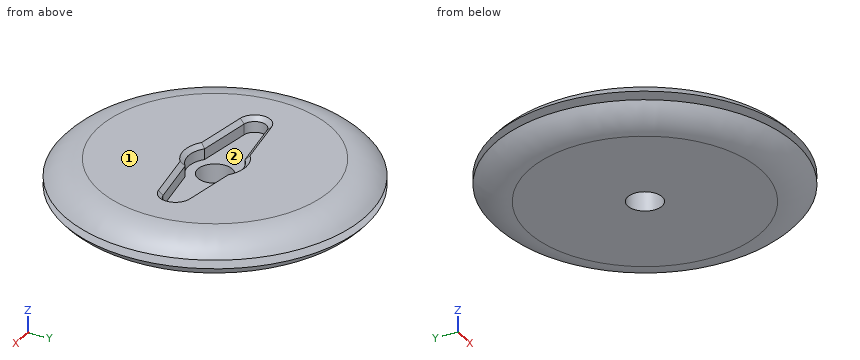
from build123d import *

# Parameters (mm, degrees)
SKETCH_1_R               = 1.5
EXTRUDE_1_DEPTH          = 2.3
SKETCH_2_R               = 4.4
EXTRUDE_2_DEPTH          = 3.2
SKETCH_3_R               = 4.4
SKETCH_3_R_2             = 3.4
SKETCH_3_R_3             = 2.75
SKETCH_3_R_4             = 1.5
CUT_EXTRUDE_1_DEPTH      = 1
BOSS_EXTRUDE1_DEPTH      = 2
BOSS_EXTRUDE1_DEPTH_BACK = 2
SKETCH1_R                = 35
INTERSECT2_OUTLINE_R     = 4.4
INTERSECT2_OUTLINE_R_2   = 3.4
INTERSECT2_OUTLINE_R_3   = 2.75
INTERSECT2_DEPTH         = 5.5
INTERSECT2_START         = 1
INTERSECT2_2_OUTLINE_R   = 4.4
INTERSECT2_2_OUTLINE_R_2 = 3.4
INTERSECT2_2_OUTLINE_R_3 = 2.75
INTERSECT2_2_OUTLINE_R_4 = 1.5
INTERSECT2_2_DEPTH       = 4.5
FILLET1_R                = 10
SKETCH2_R                = 25
BOSS_EXTRUDE2_DEPTH      = 2
SKETCH3_R                = 27
BOSS_EXTRUDE3_DEPTH      = 2
SKETCH4_R                = 6
CUT_EXTRUDE1_DEPTH       = 2
CUT_EXTRUDE3_REACH       = 52.14
SKETCH5_R                = 4
CUT_EXTRUDE4_START       = -2
CUT_EXTRUDE4_DEPTH       = 2
CHAMFER1_SIZE            = 1
CUT_EXTRUDE5_DEPTH       = 1.5


# Read off the part's stored shape, not the designer's step: Intersect2
with BuildPart() as part:
    # Эскиз1 → Бобышка-Вытянуть1 (new body)
    with BuildSketch(Plane.XY):
        with BuildLine():
            Line((-3.968626967, 4.5), (-16.888114198, 2.469689731))
            ThreePointArc((-16.888114198, 2.469689731), (-19, 0), (-16.888114198, -2.469689731))
            Line((-16.888114198, -2.469689731), (-3.968626967, -4.5))
            ThreePointArc((-3.968626967, -4.5), (0, -6), (3.968626967, -4.5))
            Line((3.968626967, -4.5), (16.888114198, -2.469689731))
            ThreePointArc((16.888114198, -2.469689731), (19, 0), (16.888114198, 2.469689731))
            Line((16.888114198, 2.469689731), (3.968626967, 4.5))
            ThreePointArc((3.968626967, 4.5), (0, 6), (-3.968626967, 4.5))
        make_face()
        Circle(SKETCH_1_R, mode=Mode.SUBTRACT)
    extrude(amount=EXTRUDE_1_DEPTH)

    # Эскиз2 → Бобышка-Вытянуть2 (add)
    with BuildSketch(Plane.XY.offset(2.3)):
        with Locations(Location((0, 0, 0), (0, 0, 180))):
            Circle(SKETCH_2_R)
        Polygon((0.333439775, 2.639447604), (0, 3.05), (-0.333439775, 2.639447604), (-0.758504156, 2.954178641), (-0.979368078, 2.473601404), (-1.469348706, 2.672735374), (-1.563759083, 2.15232973), (-2.087868673, 2.223354314), (-2.049893354, 1.695819264), (-2.575200173, 1.634271725), (-2.407225286, 1.132754236), (-2.900722375, 0.942501833), (-2.6133024, 0.498514094), (-3.043981522, 0.191511085), (-2.655176114, -0.167049522), (-2.995976115, -0.571513009), (-2.530215347, -0.822116802), (-2.75972251, -1.298626839), (-2.246271844, -1.42552746), (-2.35006539, -1.944143169), (-1.821186821, -1.939366985), (-1.792745019, -2.467501833), (-1.281669931, -2.33134895), (-1.122779886, -2.835818282), (-0.661621006, -2.576843686), (-0.382266362, -3.025949839), (0, -2.660425857), (0.382266362, -3.025949839), (0.661621006, -2.576843686), (1.122779886, -2.835818282), (1.281669931, -2.33134895), (1.792745019, -2.467501833), (1.821186821, -1.939366985), (2.35006539, -1.944143169), (2.246271844, -1.42552746), (2.75972251, -1.298626839), (2.530215347, -0.822116802), (2.995976115, -0.571513009), (2.655176114, -0.167049522), (3.043981522, 0.191511085), (2.6133024, 0.498514094), (2.900722375, 0.942501833), (2.407225286, 1.132754236), (2.575200173, 1.634271725), (2.049893354, 1.695819264), (2.087868673, 2.223354314), (1.563759083, 2.15232973), (1.469348706, 2.672735374), (0.979368078, 2.473601404), (0.758504156, 2.954178641), align=None, mode=Mode.SUBTRACT)
    extrude(amount=EXTRUDE_2_DEPTH)

    # Эскиз3 → Вырез-Вытянуть1 (cut)
    # profile 1 of 2: a face of its own
    with BuildSketch(Plane(origin=(0, 0, 0), x_dir=(-1, 0, 0), z_dir=(0, 0, -1))):
        Circle(SKETCH_3_R)
        Circle(SKETCH_3_R_2, mode=Mode.SUBTRACT)
    # profile 2 of 2: a face of its own
    with BuildSketch(Plane(origin=(0, 0, 0), x_dir=(-1, 0, 0), z_dir=(0, 0, -1))):
        Circle(SKETCH_3_R_3)
        Circle(SKETCH_3_R_4, mode=Mode.SUBTRACT)
    extrude(amount=-CUT_EXTRUDE_1_DEPTH, mode=Mode.SUBTRACT)


with BuildPart() as body_2:
    # Sketch1 → Boss-Extrude1 (new, two sides: drawn at the far end of the back side and taken through both)
    with BuildSketch(Plane(origin=(0, 0, 0), x_dir=(-1, 0, 0), z_dir=(0, 0, -1)).offset(-BOSS_EXTRUDE1_DEPTH_BACK)):
        Circle(SKETCH1_R)
    extrude(amount=BOSS_EXTRUDE1_DEPTH + BOSS_EXTRUDE1_DEPTH_BACK)


with BuildPart() as intersect2_tool:
    # Intersect2 outline → Intersect2 (new body)
    # profile 1 of 2: a face of its own
    with BuildSketch(Plane.XY):
        with BuildLine():
            ThreePointArc((3.968626967, 4.5), (0, 6), (-3.968626967, 4.5))
            Line((-3.968626967, 4.5), (-16.888114198, 2.469689731))
            ThreePointArc((-16.888114198, 2.469689731), (-19, 0), (-16.888114198, -2.469689731))
            Line((-16.888114198, -2.469689731), (-3.968626967, -4.5))
            ThreePointArc((-3.968626967, -4.5), (0, -6), (3.968626967, -4.5))
            Line((3.968626967, -4.5), (16.888114198, -2.469689731))
            ThreePointArc((16.888114198, -2.469689731), (19, 0), (16.888114198, 2.469689731))
            Line((16.888114198, 2.469689731), (3.968626967, 4.5))
        make_face()
        Circle(INTERSECT2_OUTLINE_R, mode=Mode.SUBTRACT)
    # profile 2 of 2: a face of its own
    with BuildSketch(Plane.XY):
        Circle(INTERSECT2_OUTLINE_R_2)
        Circle(INTERSECT2_OUTLINE_R_3, mode=Mode.SUBTRACT)
    extrude(amount=INTERSECT2_DEPTH)


with BuildPart() as part_1:
    add(part.part)

    # Intersect2: cut by intersect2_tool
    add(intersect2_tool.part, mode=Mode.SUBTRACT)


with BuildPart() as body_2_1:
    add(body_2.part)

    # Intersect2: cut by intersect2_tool
    add(intersect2_tool.part, mode=Mode.SUBTRACT)


with BuildPart() as intersect2_2_tool:
    # Intersect2 2 outline → Intersect2 2 (new body)
    # profile 1 of 2: a face of its own
    with BuildSketch(Plane.XY.offset(INTERSECT2_START)):
        Circle(INTERSECT2_2_OUTLINE_R)
        Circle(INTERSECT2_2_OUTLINE_R_2, mode=Mode.SUBTRACT)
    # profile 2 of 2: a face of its own
    with BuildSketch(Plane.XY.offset(INTERSECT2_START)):
        Circle(INTERSECT2_2_OUTLINE_R_3)
        Circle(INTERSECT2_2_OUTLINE_R_4, mode=Mode.SUBTRACT)
    extrude(amount=INTERSECT2_2_DEPTH)


with BuildPart() as part_2:
    add(part_1.part)

    # Intersect2 2: cut by intersect2_2_tool
    add(intersect2_2_tool.part, mode=Mode.SUBTRACT)


with BuildPart() as body_2_2:
    add(body_2_1.part)

    # Intersect2 2: cut by intersect2_2_tool
    add(intersect2_2_tool.part, mode=Mode.SUBTRACT)

    # Fillet1
    # the kernel refuses this fillet: 10 mm, written as the material it takes off along each edge
    with BuildSketch(Plane(origin=(0, 0, 2), x_dir=(-1, 0, 0), z_dir=(0, -1, 0))) as fillet1_piece_1:
        with BuildLine():
            CenterArc((27, 10), FILLET1_R, 270, 53.130102354)
            Line((27, 0), (27, -0.2))
            Line((27, -0.2), (35, -0.2))
            Line((35, -0.2), (35.2, 0))
            ThreePointArc((35.2, 0), (35.2, 2), (35.16, 3.88))
            Line((35.16, 3.88), (35, 4))
        make_face()
    revolve(axis=Axis((0, 0, 2), (0, 0, -1)), mode=Mode.SUBTRACT)


with BuildPart() as body_2_2_1:
    # Mirror9: mirrored copy
    add(body_2_2.part.mirror(Plane.XY.offset(-3)))


with BuildPart() as body_2_3:
    add(body_2_2.part)

    add(body_2_2_1.part)  # Boss-Extrude2 merges body 2 2
    # Sketch2 → Boss-Extrude2 (add)
    with BuildSketch(Plane(origin=(0, 0, -2), x_dir=(-1, 0, 0), z_dir=(0, 0, -1))):
        Circle(SKETCH2_R)
    extrude(amount=BOSS_EXTRUDE2_DEPTH)

    # Sketch3 → Boss-Extrude3 (add)
    with BuildSketch(Plane(origin=(0, 0, -8), x_dir=(-1, 0, 0), z_dir=(0, 0, -1))):
        Circle(SKETCH3_R)
    extrude(amount=-BOSS_EXTRUDE3_DEPTH)

    # Sketch4 → Cut-Extrude1 (cut)
    with BuildSketch(Plane.XY):
        Circle(SKETCH4_R)
    extrude(amount=CUT_EXTRUDE1_DEPTH, mode=Mode.SUBTRACT)

    # Sketch5 → Cut-Extrude3 (cut, up to next)
    with BuildSketch(Plane.XY, mode=Mode.PRIVATE) as cut_extrude3_sk1:
        Circle(SKETCH5_R)
    cut_extrude3_tool1 = extrude(cut_extrude3_sk1.sketch, amount=-CUT_EXTRUDE3_REACH, mode=Mode.PRIVATE) & body_2_3.part
    add(cut_extrude3_tool1.solids().sort_by_distance((0, 0, 0))[0], mode=Mode.SUBTRACT)

    # Sketch6 → Cut-Extrude4 (cut)
    with BuildSketch(Plane.XY.offset(2).offset(CUT_EXTRUDE4_START)):
        with BuildLine():
            Line((16.919163334, 2.66726491), (4.056712891, 4.68861179))
            ThreePointArc((4.056712891, 4.68861179), (0, 6.2), (-4.056712891, 4.68861179))
            Line((-4.056712891, 4.68861179), (-16.919163334, 2.66726491))
            ThreePointArc((-16.919163334, 2.66726491), (-19.2, 0), (-16.919163334, -2.66726491))
            Line((-16.919163334, -2.66726491), (-4.056712891, -4.68861179))
            ThreePointArc((-4.056712891, -4.68861179), (0, -6.2), (4.056712891, -4.68861179))
            Line((4.056712891, -4.68861179), (16.919163334, -2.66726491))
            ThreePointArc((16.919163334, -2.66726491), (19.2, 0), (16.919163334, 2.66726491))
        make_face()
    extrude(amount=CUT_EXTRUDE4_DEPTH, mode=Mode.SUBTRACT)

    # Chamfer1
    chamfer1_edges = [body_2_3.edges().sort_by_distance(p)[0] for p in [
        (0, 6.2, 2),
        (-10.487938112, 3.67793835, 2),
        (-19.2, 0, 2),
        (-10.487938112, -3.67793835, 2),
        (0, -6.2, 2),
        (10.487938112, -3.67793835, 2),
        (19.2, 0, 2),
        (10.487938112, 3.67793835, 2),
    ]]
    chamfer(chamfer1_edges, length=CHAMFER1_SIZE)

    # Sketch8 → Cut-Extrude5 (cut)
    with BuildSketch(Plane.XY):
        with BuildLine():
            Line((-4.056712891, 4.68861179), (-16.919163334, 2.66726491))
            ThreePointArc((-16.919163334, 2.66726491), (-19.2, 0), (-16.919163334, -2.66726491))
            Line((-16.919163334, -2.66726491), (-4.056712891, -4.68861179))
            ThreePointArc((-4.056712891, -4.68861179), (0, -6.2), (4.056712891, -4.68861179))
            Line((4.056712891, -4.68861179), (16.919163334, -2.66726491))
            ThreePointArc((16.919163334, -2.66726491), (19.2, 0), (16.919163334, 2.66726491))
            Line((16.919163334, 2.66726491), (4.056712891, 4.68861179))
            ThreePointArc((4.056712891, 4.68861179), (0, 6.2), (-4.056712891, 4.68861179))
        make_face()
    extrude(amount=-CUT_EXTRUDE5_DEPTH, mode=Mode.SUBTRACT)


solid = body_2_3.part
Can you work these out from the model? Positions are in its coordinate system, mm. Face numbers are marked on the shaded views. Coordinates: 2 decimals unless noted, no trailing zeros. Write each loop counter-clockwise with the first axis right and the second up, starting at its lowest first coordinate (ties: lowest second). Pieces come first, ordered by that corner, then holes. Notation, with made-up numbers: (83, -9) -> (109, -9) arc R31 cw to (109, 22) -> close; hole circle Ø7 at (36.5, -18). An arc over 180 degrees is marked (long way). Write item = value, one per line.
(1) Imagine slicing it at B-B (x = 0). Please give me the cut outline in (y, z).
Verdict:
outline = (-35, -4) arc R10 ccw to (-27, -8) -> (-4, -8) -> (-4, -1.5) -> (-6.2, -1.5) -> (-6.2, 1) -> (-7.2, 2) -> (-27, 2) arc R10 ccw to (-35, -2) -> (-25, -2) -> (-25, -4) -> close; (4, -8) -> (27, -8) arc R10 ccw to (35, -4) -> (25, -4) -> (25, -2) -> (35, -2) arc R10 ccw to (27, 2) -> (7.2, 2) -> (6.2, 1) -> (6.2, -1.5) -> (4, -1.5) -> close
(2) Imagine slicing it at C-C (z = -3). Please give me the cut outline in (x, y).
Verdict:
outline = circle Ø50 at (0, 0); hole circle Ø8 at (0, 0)
(3) If I drill on probe 1 along Y at (x, z) = (0, -3); probe 2 along Z at (x, y) = (-11, 26.5); probe 3 along Y at (x, z) = (-21, 0.25), over which ranges is the centre line in solid material (lowest first)?
Verdict:
probe_1 = -25 to -4, 4 to 25
probe_2 = -7.86 to -4, -2 to 1.86
probe_3 = -25 to 25
(4) Imagine slicing it at A-A (y = 0). Please give me the cut outline in (x, z), and give its area (3 significant figures).
Verdict:
outline = (-35, -4) arc R10 ccw to (-27, -8) -> (-4, -8) -> (-4, -1.5) -> (-19.2, -1.5) -> (-19.2, 1) -> (-20.2, 2) -> (-27, 2) arc R10 ccw to (-35, -2) -> (-25, -2) -> (-25, -4) -> close; (4, -8) -> (27, -8) arc R10 ccw to (35, -4) -> (25, -4) -> (25, -2) -> (35, -2) arc R10 ccw to (27, 2) -> (20.2, 2) -> (19.2, 1) -> (19.2, -1.5) -> (4, -1.5) -> close
area = 434 mm^2
(5) For pin 1 (2 mm diameter, centred on y = 16.5, z = 1, fed in from -X); pin 2 (1 mm diameter, centred on x = 26, y = -20.5, fed in from -Z); pin 3 (4 mm diameter, centred on x = -12, z = -0.5, fed in from -Y); pin 4 (13.5 mm diameter, centred on x = -6, y = -1.5, fed in from +Z), each with a flat end and sliding along its axis, tell me the tip position at first contact or that it passes through.
Verdict:
pin_1 = -28.68
pin_2 = -6.28
pin_3 = -33.33
pin_4 = 2
(6) Imagine slicing it at D-D (z = -7). Please give me the cut outline in (x, y), and give its area (3 significant figures).
Verdict:
outline = circle Ø62.72 at (0, 0); hole circle Ø8 at (0, 0)
area = 3,040 mm^2
(7) Thinking about a two-plate mould opening in Y: for the marked faces 1 and 2, which applies, +Y half, -Y half, draft (parallel to the pull), parting line (faces both ways), or undercut?
Verdict:
face_1 = draft
face_2 = undercut
